Here's how the part is built. I have some questions about the finished solid (model axes, mm). A direction names the side the tool comes from. Give positions to 0.01 mm unless a question says otherwise; leave off trailing zeros. Loops run counter-clockwise (first coordinate to the right, second up) from the corner with the lowest first, then second, coordinate; pieces in that order, holes last.
Q1. Thinking about a two-plate mould opening in Y: for faces 1 (the face through (24, -10, 0)), 2 (the face through (18.372, -17.364, -13.107)), which applies, pulls with the +Y half, pulls with the -Y half, needs draft (parallel to the pull), parting line crosses it, or undercut?
Q2. Suppose I cut it at D-D (z = 0). List the corners of the cut face in (x, y) for me, and give its area (3 significant figures).
Q3. Suppose I cut it at C-C (y = -32). List the corners of the cut face in (x, z) for me.
Q4. I'm going to push flat-ended pins straight in: P1, Ø2, axis at y = -34, z = 20, coming from the -X side; P2, Ø3.5, axis at x = 26, y = -11, coming from the +Z side; P3, Ø1.2, axis at x = 22.5, y = -9.5, coming from the -Z side. Where does each tip first touch, or does it pass through?
Q5. For faces 3 (the face through (-39.05, -24.65, -8.67)), 4 (the face through (22, -7, -2.5)), 5 (the face through (24.513, -15.464, 10.76)), which set-ups out of +Z, -Z, +X, -X, +Y, -Y let a thin tool reach every point of the face, with its end or its side?
Q6. Suppose I cut it at B-B (z = -30). List the corners of the cut face in (x, y) for me, and give its area (3 significant figures).
Q7. Suppose I cut it at A-A (x = 0). List the corners of the cut face in (y, z) for me.
Q8. I need wall thicknesses on probe 1 along X at (y, z) = (-18, 0); probe 2 along Y at (x, z) = (-14, 22); probe 3 along X at (y, z) = (-34, 0). Which ranges of each line are inside material? Lowest first, please.
```python
from build123d import *

# Parameters (mm, degrees)
SKETCH1_R                    = 40
BOSS_EXTRUDE1_DEPTH          = 50
CUT_EXTRUDE1_DEPTH           = 20
SKETCH2_W                    = 5.5
SKETCH2_H                    = 5.2
CUT_REVOLVE1_ANGLE           = 30
CUT_REVOLVE1_OTHER_WAY_ANGLE = 30
SHELL1_START                 = -46
SHELL1_OUTLINE_R             = 36
SHELL1_DEPTH                 = 26
SHELL1_START_2               = -20
SHELL1_2_OUTLINE_R           = 36
SHELL1_2_DEPTH               = 16
SHELL1_START_3               = -10.8
SHELL1_3_DEPTH               = 6.8


# Read off the part's stored shape, not the designer's step: Shell1
with BuildPart() as part:
    # Sketch1 → Boss-Extrude1 (new body)
    with BuildSketch(Plane(origin=(0, 0, 0), x_dir=(1, 0, 0), z_dir=(0, 1, 0))):
        with Locations(Location((0, 0, 0), (0, 0, 270))):
            Circle(SKETCH1_R)
    extrude(amount=-BOSS_EXTRUDE1_DEPTH)

    # Sketch1<3> → Cut-Extrude1 (cut)
    with BuildSketch(Plane(origin=(0, 0, 0), x_dir=(1, 0, 0), z_dir=(0, 1, 0))):
        with BuildLine():
            Line((19.843134833, 2.5), (23.869436525, 2.5))
            ThreePointArc((23.869436525, 2.5), (24, 0), (23.869436525, -2.5))
            Line((23.869436525, -2.5), (19.843134833, -2.5))
            ThreePointArc((19.843134833, -2.5), (0, -20), (-19.843134833, -2.5))
            Line((-19.843134833, -2.5), (-23.869436525, -2.5))
            ThreePointArc((-23.869436525, -2.5), (-24, 0), (-23.869436525, 2.5))
            Line((-23.869436525, 2.5), (-19.843134833, 2.5))
            ThreePointArc((-19.843134833, 2.5), (0, 20), (19.843134833, 2.5))
        make_face()
    extrude(amount=-CUT_EXTRUDE1_DEPTH, mode=Mode.SUBTRACT)

    # Sketch2 → Cut-Revolve1 (revolve, cut)
    with BuildSketch(Plane.XY.offset(-2.5)):
        with Locations((-21.119436525, -17.4)):
            Rectangle(SKETCH2_W, SKETCH2_H)
        with Locations((21.119436525, -17.4)):
            Rectangle(SKETCH2_W, SKETCH2_H)
    revolve(axis=Axis((0, -29.434320881, -2.5), (0, 1, 0)), revolution_arc=CUT_REVOLVE1_ANGLE, mode=Mode.SUBTRACT)

    # Sketch2 → Cut-Revolve1 other way (revolve, cut)
    with BuildSketch(Plane.XY.offset(-2.5)):
        with Locations((-21.119436525, -17.4)):
            Rectangle(SKETCH2_W, SKETCH2_H)
        with Locations((21.119436525, -17.4)):
            Rectangle(SKETCH2_W, SKETCH2_H)
    revolve(axis=Axis((0, -29.434320881, -2.5), (0, -1, 0)), revolution_arc=CUT_REVOLVE1_OTHER_WAY_ANGLE, mode=Mode.SUBTRACT)

    # Shell1 outline → Shell1 (cut)
    with BuildSketch(Plane(origin=(0, 0, 0), x_dir=(1, 0, 0), z_dir=(0, 1, 0)).offset(SHELL1_START)):
        Circle(SHELL1_OUTLINE_R)
    extrude(amount=SHELL1_DEPTH, mode=Mode.SUBTRACT)

    # Shell1 2 outline → Shell1 2 (cut)
    with BuildSketch(Plane(origin=(0, 0, 0), x_dir=(1, 0, 0), z_dir=(0, 1, 0)).offset(SHELL1_START_2)):
        Circle(SHELL1_2_OUTLINE_R)
        with BuildLine():
            Line((-26.376229681, -6.5), (-27.235087663, -6.5))
            ThreePointArc((-27.235087663, -6.5), (-27.933967525, -1.921837216), (-27.86865358, 2.708901561))
            ThreePointArc((-27.86865358, 2.708901561), (-26.29664821, 11.729939607), (-21.885751383, 19.754546606))
            Line((-21.885751383, 19.754546606), (-17.004628173, 16.936428806))
            ThreePointArc((-17.004628173, 16.936428806), (0, 24), (17.004628173, 16.936428806))
            Line((17.004628173, 16.936428806), (21.885751383, 19.754546606))
            ThreePointArc((21.885751383, 19.754546606), (26.29664821, 11.729939607), (27.86865358, 2.708901561))
            ThreePointArc((27.86865358, 2.708901561), (27.933967525, -1.921837216), (27.235087663, -6.5))
            Line((27.235087663, -6.5), (26.376229681, -6.5))
            ThreePointArc((26.376229681, -6.5), (24.481402921, -10.817897852), (21.885751383, -14.754546606))
            Line((21.885751383, -14.754546606), (19.806304482, -13.553977378))
            ThreePointArc((19.806304482, -13.553977378), (0, -24), (-19.806304482, -13.553977378))
            Line((-19.806304482, -13.553977378), (-21.885751383, -14.754546606))
            ThreePointArc((-21.885751383, -14.754546606), (-24.481402921, -10.817897852), (-26.376229681, -6.5))
        make_face(mode=Mode.SUBTRACT)
    extrude(amount=SHELL1_2_DEPTH, mode=Mode.SUBTRACT)

    # Shell1 3 outline → Shell1 3 (cut)
    with BuildSketch(Plane(origin=(0, 0, 0), x_dir=(1, 0, 0), z_dir=(0, 1, 0)).offset(SHELL1_START_3)):
        with BuildLine():
            Line((-23.103030104, -6.5), (-26.376229681, -6.5))
            ThreePointArc((-26.376229681, -6.5), (-24.481402921, -10.817897852), (-21.885751383, -14.754546606))
            Line((-21.885751383, -14.754546606), (-19.806304482, -13.553977378))
            ThreePointArc((-19.806304482, -13.553977378), (-21.742640085, -10.161574786), (-23.103030104, -6.5))
        make_face()
        with BuildLine():
            ThreePointArc((-21.885751383, 19.754546606), (-26.29664821, 11.729939607), (-27.86865358, 2.708901561))
            ThreePointArc((-27.86865358, 2.708901561), (-27.616999866, 4.615335138), (-27.235087663, 6.5))
            Line((-27.235087663, 6.5), (-23.103030104, 6.5))
            ThreePointArc((-23.103030104, 6.5), (-20.721626979, 12.108434057), (-17.004628173, 16.936428806))
            Line((-17.004628173, 16.936428806), (-21.885751383, 19.754546606))
        make_face()
        with BuildLine():
            ThreePointArc((23.103030104, -6.5), (21.742640085, -10.161574786), (19.806304482, -13.553977378))
            Line((19.806304482, -13.553977378), (21.885751383, -14.754546606))
            ThreePointArc((21.885751383, -14.754546606), (24.481402921, -10.817897852), (26.376229681, -6.5))
            Line((26.376229681, -6.5), (23.103030104, -6.5))
        make_face()
        with BuildLine():
            Line((21.885751383, 19.754546606), (17.004628173, 16.936428806))
            ThreePointArc((17.004628173, 16.936428806), (20.721626979, 12.108434057), (23.103030104, 6.5))
            Line((23.103030104, 6.5), (27.235087663, 6.5))
            ThreePointArc((27.235087663, 6.5), (27.616999866, 4.615335138), (27.86865358, 2.708901561))
            ThreePointArc((27.86865358, 2.708901561), (26.29664821, 11.729939607), (21.885751383, 19.754546606))
        make_face()
    extrude(amount=SHELL1_3_DEPTH, mode=Mode.SUBTRACT)


solid = part.part
```
Solutions:
1. face 1: needs draft
1. face 2: undercut
2. outline: (-40, -50) - (40, -50) - (40, 0) - (24, 0) - (24, -20) - (28, -20) - (28, -4) - (36, -4) - (36, -46) - (-36, -46) - (-36, -4) - (-28, -4) - (-28, -20) - (-24, -20) - (-24, 0) - (-40, 0) - close
2. area: 912 mm2
3. outline: circle Ø80 at (0, 0); hole circle Ø72 at (0, 0)
4. P1: stops at x = -35.2
4. P2: stops at z = 31.81
4. P3: stops at z = -33.47
5. face 3: +Y, -Y
5. face 4: +Y
5. face 5: none
6. outline: (-26.46, -50) - (26.46, -50) - (26.46, 0) - (-26.46, 0) - close; hole (-19.9, -46) - (19.9, -46) - (19.9, -4) - (-19.9, -4) - close
6. area: 974 mm2
7. outline: (-50, -40) - (0, -40) - (0, -20) - (-20, -20) - (-20, -24) - (-4, -24) - (-4, -36) - (-46, -36) - (-46, 36) - (-4, 36) - (-4, 24) - (-20, 24) - (-20, 20) - (0, 20) - (0, 40) - (-50, 40) - close
8. probe 1: x = -40 to -36, -28 to -24, 24 to 28, 36 to 40
8. probe 2: y = -50 to -46, -4 to 0
8. probe 3: x = -40 to -36, 36 to 40
